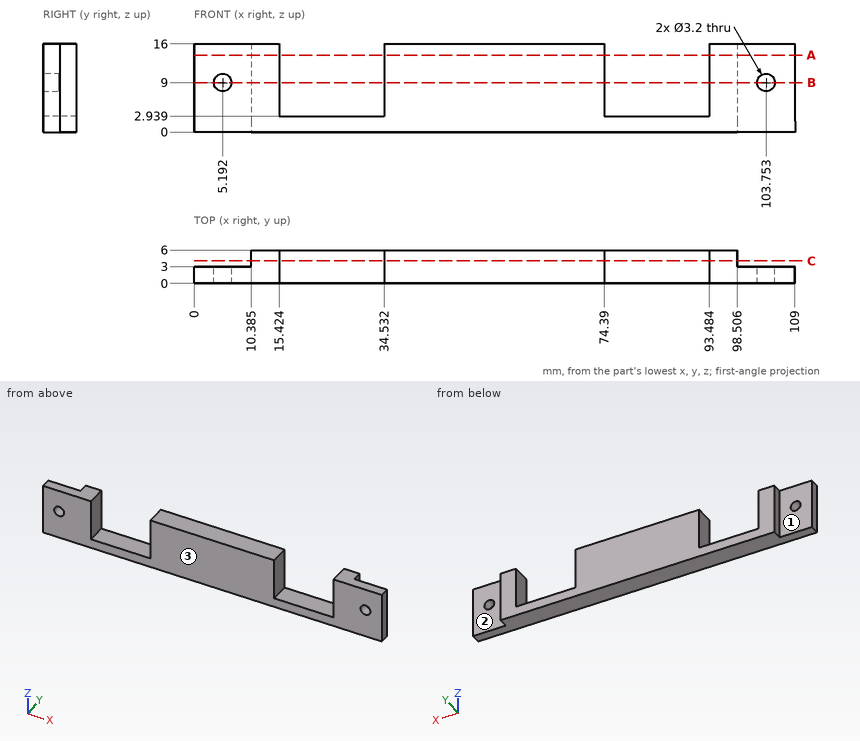
Could you check a few things on this drawing? It's one solid part, dimensions in mm from its lowest x, y, z. A direction names the side the tool comes from. Coordinates: 2 decimals unless noted, no trailing zeros. Write each loop counter-clockwise with the first axis right and the second up, starting at its lowest first coordinate (ties: lowest second). Pieces come first, ordered by that corner, then holes. Notation, with made-up numbers: (14, 14.25) - (67, 14.25) arc R3 cw to (67, 19.25) - close; hole circle Ø3 at (-23.5, 32.5). An arc over 180 degrees is marked (long way). Write item = value, one per line.
1) Suppose I cut it at A-A on z = 14. Please give me the cut outline in (x, y) (1 decimal).
Result set:
outline = (0, 0) - (15.4, 0) - (15.4, 6) - (10.4, 6) - (10.4, 3) - (0, 3) - close; (34.5, 0) - (74.4, 0) - (74.4, 6) - (34.5, 6) - close; (93.5, 0) - (109, 0) - (109, 3) - (98.5, 3) - (98.5, 6) - (93.5, 6) - close
2) Please list where these lines run through material, in increasing order: line 1 (X direction, y = 3.3, z = 14.75) (1 decimal); line 2 (X direction, y = 1.45, z = 9) (1 decimal); line 3 (X direction, y = 0.95, z = 12.75) (1 decimal). Write a range as [from, to].
Result set:
line_1 = [10.4, 15.4], [34.5, 74.4], [93.5, 98.5]
line_2 = [0, 3.6], [6.8, 15.4], [34.5, 74.4], [93.5, 102.2], [105.4, 109]
line_3 = [0, 15.4], [34.5, 74.4], [93.5, 109]
3) Suppose I cut it at B-B on z = 9. Please give me the cut outline in (x, y) (1 decimal), plus the area to 3 significant figures.
Result set:
outline = (0, 0) - (3.6, 0) - (3.6, 3) - (0, 3) - close; (6.8, 0) - (15.4, 0) - (15.4, 6) - (10.4, 6) - (10.4, 3) - (6.8, 3) - close; (34.5, 0) - (74.4, 0) - (74.4, 6) - (34.5, 6) - close; (93.5, 0) - (102.2, 0) - (102.2, 3) - (98.5, 3) - (98.5, 6) - (93.5, 6) - close; (105.4, 0) - (109, 0) - (109, 3) - (105.4, 3) - close
area = 343 mm2
4) Suppose I cut it at C-C on y = 4.05. Please give me the cut outline in (x, z) (1 decimal), plus the area to 3 significant figures.
Result set:
outline = (10.4, 0) - (98.5, 0) - (98.5, 16) - (93.5, 16) - (93.5, 2.9) - (74.4, 2.9) - (74.4, 16) - (34.5, 16) - (34.5, 2.9) - (15.4, 2.9) - (15.4, 16) - (10.4, 16) - close
area = 911 mm2
5) Will these pins go through, and if not, where does the flat tip stop? pin 1 Ø3 at (x, z) = (5.19, 9) entering from -Y; pin 2 Ø1.5 at (y, z) = (4, 5.5) entering from +X; pin 3 Ø3 at (x, z) = (7, 4.5) entering from +Y.
Result set:
pin_1 = through
pin_2 = 98.51
pin_3 = 3
6) For the marked faces 1, 2 and 3, which set-ups out of +Z, -Z, +X, -X, +Y, -Y let a thin tool reach every point of the face, with its end or its side?
Result set:
face_1 = +Z, -Z, -X, +Y
face_2 = +Z, -Z, +X, +Y
face_3 = +Z, -Z, +X, -X, -Y
